from build123d import *

# Parameters (mm, degrees)
SKETCH1_W                   = 25.4
SKETCH1_H                   = 25.4
BOSS_EXTRUDE1_DEPTH         = 101.6
FILLET1_R                   = 1.5875
HOLE1_OUTLINE_R             = 2.5527
HOLE1_DEPTH                 = 101.6
SKETCH7_W                   = 6.5278
SKETCH7_H                   = 2.2352
CUT_EXTRUDE2_DEPTH          = 101.6
FILLET4_R                   = 0.396875
CIRPATTERN2_DEPTH           = 101.6
F_1_4_20_TAPPED_HOLE1_D     = 5.1054
F_1_4_20_TAPPED_HOLE1_DEPTH = 6.35
F_1_4_20_TAPPED_HOLE1_TIP   = 1.533816902


# Read off the part's stored shape, not the designer's step: Hole1, CirPattern2
with BuildPart() as part:
    # Sketch1 → Boss-Extrude1 (new body)
    with BuildSketch(Plane.XY):
        Rectangle(SKETCH1_W, SKETCH1_H)
    extrude(amount=BOSS_EXTRUDE1_DEPTH)

    # Fillet1
    fillet1_edges = [part.edges().sort_by_distance(p)[0] for p in [
        (12.7, -12.7, 50.8),
        (-12.7, -12.7, 50.8),
        (-12.7, 12.7, 50.8),
        (12.7, 12.7, 50.8),
    ]]
    fillet(fillet1_edges, radius=FILLET1_R)

    # Hole1 outline → Hole1 (cut)
    with BuildSketch(Plane.XY):
        with Locations((0, -0.048792482)):
            Circle(HOLE1_OUTLINE_R)
    extrude(amount=HOLE1_DEPTH, mode=Mode.SUBTRACT)

    # Sketch7 → Cut-Extrude2 (cut)
    with BuildSketch(Plane.XY.offset(101.6)):
        with Locations((0, 11.5824)):
            Rectangle(SKETCH7_W, SKETCH7_H)
        Polygon((-3.175, 4.5212), (-7.3025, 10.4648), (7.3025, 10.4648), (3.175, 4.5212), align=None)
    extrude(amount=-CUT_EXTRUDE2_DEPTH, mode=Mode.SUBTRACT)

    # Fillet4
    fillet4_edges = [part.edges().sort_by_distance(p)[0] for p in [
        (-3.2639, 10.4648, 50.8),
        (-3.2639, 12.7, 50.8),
        (3.2639, 12.7, 50.8),
        (3.2639, 10.4648, 50.8),
    ]]
    fillet(fillet4_edges, radius=FILLET4_R)

    # CirPattern2 outline → CirPattern2 (cut)
    with BuildSketch(Plane.XY):
        with BuildLine():
            ThreePointArc((-3.660775, -10.562384964), (-3.380141996, -10.67862696), (-3.2639, -10.959259964))
            Line((-3.2639, -10.959259964), (-3.2639, -12.7))
            Line((-3.2639, -12.7), (3.2639, -12.7))
            Line((3.2639, -12.7), (3.2639, -10.959259964))
            ThreePointArc((3.2639, -10.959259964), (3.380141996, -10.67862696), (3.660775, -10.562384964))
            Line((3.660775, -10.562384964), (7.3025, -10.562384964))
            Line((7.3025, -10.562384964), (3.175, -4.618784964))
            Line((3.175, -4.618784964), (-3.175, -4.618784964))
            Line((-3.175, -4.618784964), (-7.3025, -10.562384964))
            Line((-7.3025, -10.562384964), (-3.660775, -10.562384964))
        make_face()
        with BuildLine():
            Line((-12.7, -3.312692482), (-10.910467482, -3.312692482))
            ThreePointArc((-10.910467482, -3.312692482), (-10.629834478, -3.428934478), (-10.513592482, -3.709567482))
            Line((-10.513592482, -3.709567482), (-10.513592482, -7.351292482))
            Line((-10.513592482, -7.351292482), (-4.569992482, -3.223792482))
            Line((-4.569992482, -3.223792482), (-4.569992482, 3.126207518))
            Line((-4.569992482, 3.126207518), (-10.513592482, 7.253707518))
            Line((-10.513592482, 7.253707518), (-10.513592482, 3.611982518))
            ThreePointArc((-10.513592482, 3.611982518), (-10.629834478, 3.331349514), (-10.910467482, 3.215107518))
            Line((-10.910467482, 3.215107518), (-12.7, 3.215107518))
            Line((-12.7, 3.215107518), (-12.7, -3.312692482))
        make_face()
        with BuildLine():
            ThreePointArc((10.513592482, -3.709567482), (10.629834478, -3.428934478), (10.910467482, -3.312692482))
            Line((10.910467482, -3.312692482), (12.7, -3.312692482))
            Line((12.7, -3.312692482), (12.7, 3.215107518))
            Line((12.7, 3.215107518), (10.910467482, 3.215107518))
            ThreePointArc((10.910467482, 3.215107518), (10.629834478, 3.331349514), (10.513592482, 3.611982518))
            Line((10.513592482, 3.611982518), (10.513592482, 7.253707518))
            Line((10.513592482, 7.253707518), (4.569992482, 3.126207518))
            Line((4.569992482, 3.126207518), (4.569992482, -3.223792482))
            Line((4.569992482, -3.223792482), (10.513592482, -7.351292482))
            Line((10.513592482, -7.351292482), (10.513592482, -3.709567482))
        make_face()
    extrude(amount=CIRPATTERN2_DEPTH, mode=Mode.SUBTRACT)

    # 1/4-20 Tapped Hole1
    with Locations(Plane(origin=(0, -0.048792482, 101.6), x_dir=(1, 0, 0), z_dir=(0, 0, 1))):
        with Locations((0, 0)):
            Hole(F_1_4_20_TAPPED_HOLE1_D / 2, depth=F_1_4_20_TAPPED_HOLE1_DEPTH)
            with Locations((0, 0, -(F_1_4_20_TAPPED_HOLE1_DEPTH + F_1_4_20_TAPPED_HOLE1_TIP / 2))):  # 118° drill point
                Cone(0, F_1_4_20_TAPPED_HOLE1_D / 2, F_1_4_20_TAPPED_HOLE1_TIP, mode=Mode.SUBTRACT)


solid = part.part
Build history of the part. All positions in model axes, mm. A direction names the side the tool comes from. Round coordinates to 2 decimals unless told otherwise and drop trailing zeros. Order: outer loops, then holes, each group sorted by start corner. A loop starts at its lowest first (then second) coordinate and runs counter-clockwise, first axis right, second up. Notation, with made-up numbers: M 79.5,-10.75 L 124.5,-10.75 A22 cw 124.5,20.25 Z; hole C 32,60.5 d10. An arc over 180 degrees is marked long. Use CSV: the item, a comma, the result in double quotes. Start each with the question number.
(1) Flat gauge pins, fed straight in: P1, Ø1.9, axis at x = 0.5, z = 71, coming from the -Y side; P2, Ø1.5, axis at y = -2.5, z = 41.5, coming from the -X side; P3, Ø3, axis at x = 1.5, z = 69.5, coming from the +Y side. Where does each tip first touch, or does it go through?
(2) Tool access for faces 1 (the face through (7.583, 5.219, 50.089)), 2 (the face through (0, 4.521, 52)), 3 (the face through (-4.57, 0, 50)): list every direction of +Z, -Z, +X, -X, +Y, -Y with a clear straight run to the whole face (end or side of a thin tool).
(3) Drill centre lines: probe 1 along Y at (x, z) = (0, 50); probe 2 along X at (y, z) = (-6.5, 70.5); probe 3 along X at (y, z) = (-11.25, 21). Where is each one in solid material? Low to high.
(4) Cut at A-A on x = 0. List the corners of the cut face in (y, z).
(5) Cut at C-C on x = 8.75. List the corners of the cut face in (y, z), then the cut area to 3 significant figures.
(6) Cut at B-B on y = 6.25. List the corners of the cut face in (x, z), then the cut area to 3 significant figures.
Findings:
1,P1,"stops at y = -4.62"
1,P2,"stops at x = -4.61"
1,P3,"stops at y = 4.52"
2,face 1,"+Z, -Z"
2,face 2,"+Z, -Z, +Y"
2,face 3,"+Z, -Z, -X"
3,probe 1,"y = -4.62 to -2.6, 2.5 to 4.52"
3,probe 2,"x = -12.7 to -10.51, -9.29 to -4.48, 4.48 to 9.29, 10.51 to 12.7"
3,probe 3,"x = -12.69 to -3.26, 3.26 to 12.69"
4,outline,"M -4.62,0 L -2.6,0 L -2.6,101.6 L -4.62,101.6 Z; M 2.5,0 L 4.52,0 L 4.52,101.6 L 2.5,101.6 Z"
5,outline,"M -12.7,0 L -6.13,0 L -6.13,101.6 L -12.7,101.6 Z; M 6.03,0 L 12.7,0 L 12.7,101.6 L 6.03,101.6 Z"
5,area,"1,350 mm^2"
6,outline,"M -12.7,0 L -10.51,0 L -10.51,101.6 L -12.7,101.6 Z; M -9.07,0 L -4.38,0 L -4.38,101.6 L -9.07,101.6 Z; M 4.38,0 L 9.07,0 L 9.07,101.6 L 4.38,101.6 Z; M 10.51,0 L 12.7,0 L 12.7,101.6 L 10.51,101.6 Z"
6,area,"1,400 mm^2"
